Part model, mm, in its own coordinate system. Face numbers are marked on the shaded views. A direction names the side the tool comes from. Coordinates: 2 decimals unless noted, no trailing zeros. Loops run counter-clockwise (first coordinate to the right, second up) from the corner with the lowest first, then second, coordinate; pieces in that order, holes last. Notation, with made-up numbers: (1, 84.25) - (46, 84.25) arc R7 ccw to (46, 89.25) - close; hole circle Ø11 at (75, -27.5). An arc over 180 degrees is marked (long way). One line per question, with ' | ' between items. Start each with the question number.
Autodesk Inventor part; units mm, degrees
ref_plane "YZ Plane" through (0, 0, 0) normal (1, 0, 0) x (0, 1, 0)
ref_plane "XZ Plane" through (0, 0, 0) normal (0, 1, 0) x (-1, 0, 0)
ref_plane "XY Plane" through (0, 0, 0) normal (0, 0, 1) x (1, 0, 0)
sketch "Sketch1" plane through (0, 0, 0) normal (0, 1, 0) x (-1, 0, 0)
  circle A0 centre (0, 0) radius 17.5
  circle A1 centre (0, 0) radius 7.5
  dimension "d0" = 35
  dimension "d1" = 15
extrude "Extrusion1" add sketch "Sketch1" along normal blind 26
sketch "Sketch2" plane through (0, 0, 0) normal (0, -1, 0) x (1, 0, 0)
  circle A0 centre (0, 0) radius 7.5
extrude "Extrusion2" add sketch "Sketch2" along normal blind 21 and the other way blind 47
fillet "Fillet1" radius 2 4 edges at (17.5, 26, 0) (17.5, 0, 0) (-7.5, 47, 0) (-7.5, -21, 0)
properties part number "Amostra_v1"
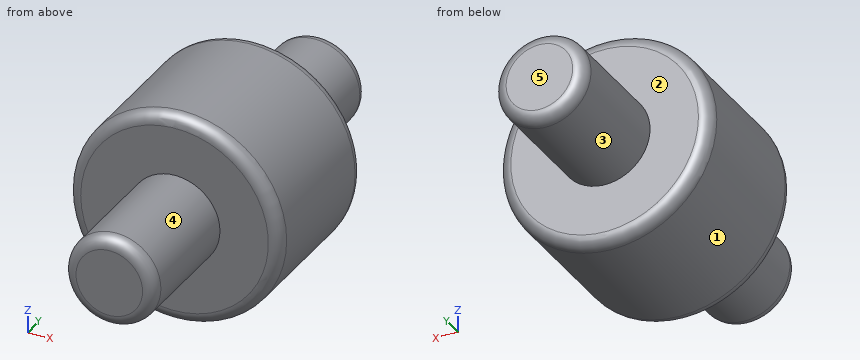
1) Wall check: line 1 along Y through (x, z) = (-7.5, 9); line 2 along Z through (x, y) = (-5.5, 40); line 3 along Z through (x, y) = (-11, 20). Give the ranges that are in metal, low to high. Write a range as [from, to].
2) Mould opens along X. For the marked faces 1 and 2 say: +X half, -X half, draft (parallel to the pull), parting line (faces both ways), or undercut.
3) Pin check, flat tips, straight feed: pin 1 Ø12 at (y, z) = (-7.5, -2) entering from -X; pin 2 Ø5 at (x, z) = (13, 0) entering from +Y; pin 3 Ø6 at (x, y) = (12.5, 16.5) entering from -Z. Stop position of each tip, or through.
4) Tool access for the marked faces 3, 4 and 5: list every direction of +Z, -Z, +X, -X, +Y, -Y with a clear straight run to the whole face (end or side of a thin tool).
5) Band-saw the part on D-D on y = -7. List the corners of the cut face in (x, z).
6) Band-saw the part on B-B on x = 0. List the corners of the cut face in (y, z), then the cut area to 3 significant figures.
7) Band-saw the part on C-C on y = 9.5. List the corners of the cut face in (x, z), then the cut area to 3 significant figures.
8) Band-saw the part on A-A on z = 0. List the corners of the cut face in (x, y).
Values found:
1) line 1: [0, 26] | line 2: [-5.1, 5.1] | line 3: [-13.61, 13.61]
2) face 1: parting line | face 2: draft
3) pin 1: x = -7.5 | pin 2: y = 26 | pin 3: z = -14.7
4) face 3: +Y | face 4: -Y | face 5: +Z, -Z, +X, -X, +Y
5) outline: circle Ø15 at (0, 0)
6) outline: (-21, -5.5) arc R2 ccw to (-19, -7.5) - (0, -7.5) - (0, -15.5) arc R2 ccw to (2, -17.5) - (24, -17.5) arc R2 ccw to (26, -15.5) - (26, -7.5) - (45, -7.5) arc R2 ccw to (47, -5.5) - (47, 5.5) arc R2 ccw to (45, 7.5) - (26, 7.5) - (26, 15.5) arc R2 ccw to (24, 17.5) - (2, 17.5) arc R2 ccw to (0, 15.5) - (0, 7.5) - (-19, 7.5) arc R2 ccw to (-21, 5.5) - close | area: 1,530 mm²
7) outline: circle Ø35 at (0, 0) | area: 962 mm²
8) outline: (-17.5, 2) arc R2 ccw to (-15.5, 0) - (-7.5, 0) - (-7.5, -19) arc R2 ccw to (-5.5, -21) - (5.5, -21) arc R2 ccw to (7.5, -19) - (7.5, 0) - (15.5, 0) arc R2 ccw to (17.5, 2) - (17.5, 24) arc R2 ccw to (15.5, 26) - (7.5, 26) - (7.5, 45) arc R2 ccw to (5.5, 47) - (-5.5, 47) arc R2 ccw to (-7.5, 45) - (-7.5, 26) - (-15.5, 26) arc R2 ccw to (-17.5, 24) - close
